Autodesk Inventor part; units mm, degrees
ref_plane "YZ Plane" through (0, 0, 0) normal (1, 0, 0) x (0, 1, 0)
ref_plane "XZ Plane" through (0, 0, 0) normal (0, 1, 0) x (-1, 0, 0)
ref_plane "XY Plane" through (0, 0, 0) normal (0, 0, 1) x (1, 0, 0)
sketch "Boceto1" plane through (0, 0, 0) normal (0, 0, 1) x (1, 0, 0)
  circle A0 centre (0, 0) radius 10
  circle A1 centre (100, 0) radius 10
  circle A2 centre (0, 0) radius 12.5
  circle A3 centre (100, 0) radius 12.5
  line L0 (0, 12.5) -> (100, 12.5)
  line L1 (0, -12.5) -> (100, -12.5)
  dimension "d0" = 20
  dimension "d1" = 20
  dimension "d2" = 25
  dimension "d3" = 25
  dimension "d4" = 100
extrude "Extrusión1" add sketch "Boceto1" along normal blind 30
properties part number "codo"
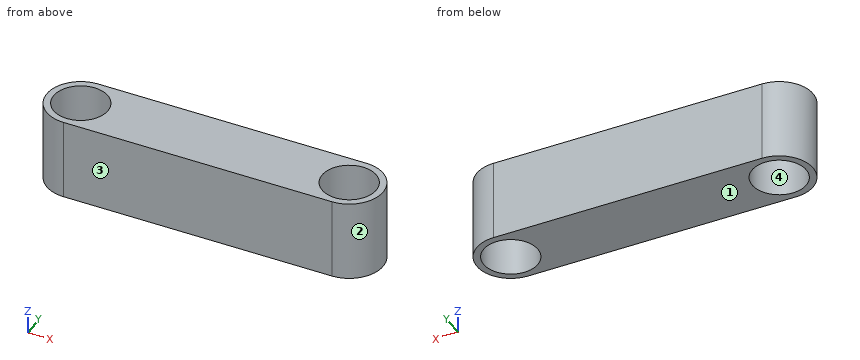
Check sheet for the modelled part. Datum: model origin and axes. Units: mm. Face numbers are marked on the shaded views. Coordinates: 2 decimals unless noted, no trailing zeros. Write each loop counter-clockwise with the first axis right and the second up, starting at its lowest first coordinate (ties: lowest second). Pieces come first, ordered by that corner, then holes.
Item 1: Cross-section at B-B on z = 11.5. Record the boundary of the cut face in (x, y), then the cut area to 3 significant figures.
Numbers:
outline: (0, -12.5) - (100, -12.5) arc R12.5 ccw to (100, 12.5) - (0, 12.5) arc R12.5 ccw to start; hole circle Ø20 at (0, 0); hole circle Ø20 at (100, 0)
area: 2,360 mm2
Item 2: Mould release check, pull along Y, two halves, no side actions. Record for the marked faces 1, 2, 3 and 4: released by +Y, released by -Y, zero draft, split by the parting line, or undercut.
Numbers:
face 1: zero draft
face 2: split by the parting line
face 3: released by -Y
face 4: undercut
Item 3: Cross-section at C-C on y = -6.5. Record the boundary of the cut face in (x, z), then the cut area to 3 significant figures.
Numbers:
outline: (-10.68, 0) - (-7.6, 0) - (-7.6, 30) - (-10.68, 30) - close; (7.6, 0) - (92.4, 0) - (92.4, 30) - (7.6, 30) - close; (107.6, 0) - (110.68, 0) - (110.68, 30) - (107.6, 30) - close
area: 2,730 mm2
Item 4: Scan lines: probe 1 along X at (y, z) = (4, 21); probe 2 along X at (y, z) = (-3.25, 26); probe 3 along Y at (x, z) = (-1, 19). Record each from-to range of solid material in increasing order.
Numbers:
probe 1: x = -11.84 to -9.17, 9.17 to 90.83, 109.17 to 111.84
probe 2: x = -12.07 to -9.46, 9.46 to 90.54, 109.46 to 112.07
probe 3: y = -12.46 to -9.95, 9.95 to 12.46
Item 5: Depth check by flat-ended pin: pin 1 Ø10 at (y, z) = (-6.5, 24.5) entering from -X; pin 2 Ø5 at (y, z) = (6.5, 20.5) entering from +X. Enter the tip coordinate at first touch or a pass-through.
Numbers:
pin 1: stops at x = -12.41
pin 2: stops at x = 111.84
Item 6: Cross-section at A-A on y = 0. Record the boundary of the cut face in (x, z).
Numbers:
outline: (-12.5, 0) - (-10, 0) - (-10, 30) - (-12.5, 30) - close; (10, 0) - (90, 0) - (90, 30) - (10, 30) - close; (110, 0) - (112.5, 0) - (112.5, 30) - (110, 30) - close
